```python
from build123d import *

# Parameters (mm, degrees)
SKETCH2_W           = 304.8
SKETCH2_H           = 17.78
BOSS_EXTRUDE1_DEPTH = 152.4
SKETCH3_W           = 121.604136641
SKETCH3_H           = 12.7
CUT_EXTRUDE1_DEPTH  = 305.8
CUT_EXTRUDE2_DEPTH  = 203.2
BOSS_EXTRUDE6_DEPTH = 63.5
BOSS_EXTRUDE8_DEPTH = 76.2
BOSS_EXTRUDE9_DEPTH = 69.163311
CUT_EXTRUDE4_REACH  = 230.6
SKETCH14_W          = 31.75
SKETCH14_H          = 203.2
CUT_EXTRUDE5_DEPTH  = 116.484487595
SKETCH15_W          = 69.163311332
SKETCH15_H          = 50.8
CUT_EXTRUDE6_DEPTH  = 12.7


with BuildPart() as part:
    # Sketch2 → Boss-Extrude1 (new body)
    with BuildSketch(Plane.XY):
        with Locations((152.4, 8.89)):
            Rectangle(SKETCH2_W, SKETCH2_H)
    extrude(amount=BOSS_EXTRUDE1_DEPTH)

    # Sketch3 → Cut-Extrude1 (cut, through all)
    with BuildSketch(Plane(origin=(304.8, 0, 0), x_dir=(0, 0, -1), z_dir=(1, 0, 0))):
        Polygon((-152.4, 17.78), (-152.4, 0), (-121.604136641, 17.78), align=None)
        with Locations((-60.802068321, 11.43)):
            Rectangle(SKETCH3_W, SKETCH3_H)
    extrude(amount=-CUT_EXTRUDE1_DEPTH, mode=Mode.SUBTRACT)

    # Sketch4 → Cut-Extrude2 (cut)
    with BuildSketch(Plane(origin=(0, 5.08, 0), x_dir=(1, 0, 0), z_dir=(0, 1, 0))):
        Polygon((0, 0), (0, -112.812583018), (117.818344334, 0), align=None)
        Polygon((304.8, 0), (186.981655666, 0), (304.8, -112.812583018), align=None)
    extrude(amount=-CUT_EXTRUDE2_DEPTH, mode=Mode.SUBTRACT)

    # Sketch5 → Boss-Extrude6 (add)
    with BuildSketch(Plane(origin=(0, 5.08, 0), x_dir=(1, 0, 0), z_dir=(0, 1, 0))):
        Polygon((127, 0), (117.818344334, 0), (0, -112.812583018), (0, -121.604136641), (12.7, -121.604136641), align=None)
        Polygon((177.8, 0), (186.981655666, 0), (304.8, -112.812583018), (304.8, -121.604136641), (292.1, -121.604136641), align=None)
    extrude(amount=BOSS_EXTRUDE6_DEPTH)

    # Sketch8 → Boss-Extrude8 (add)
    with BuildSketch(Plane(origin=(0, 0, 0), x_dir=(-1, 0, 0), z_dir=(0, 0, -1))):
        Polygon((-186.981655666, 68.58), (-186.981655666, 0), (-117.818344334, 0), (-117.818344334, 68.58), (-127, 68.58), (-127, 5.08), (-177.8, 5.08), (-177.8, 68.58), align=None)
    extrude(amount=BOSS_EXTRUDE8_DEPTH)

    # Sketch10 → Boss-Extrude9 (add)
    with BuildSketch(Plane(origin=(186.981655666, 0, 0), x_dir=(0, 0, -1), z_dir=(1, 0, 0))):
        Polygon((6.35, 0), (0, 0), (127, 219.970452561), (133.35, 219.970452561), align=None)
    extrude(amount=-BOSS_EXTRUDE9_DEPTH)

    # Cut-Extrude4: up to this face of the body (flat: up to its plane)
    cut_extrude4_end = Plane(part.part.faces().sort_by_distance((152.400000127, 118.969659324, -75.037164836))[0])
    # Sketch12 → Cut-Extrude4 (cut, up to the picked face)
    with BuildSketch(Plane(origin=(0, 0, -76.2), x_dir=(-1, 0, 0), z_dir=(0, 0, -1)), mode=Mode.PRIVATE) as cut_extrude4_sk1:
        Polygon((-186.981655666, 0), (-186.981655666, 68.58), (-177.8, 68.58), (-177.8, 5.08), (-127, 5.08), (-127, 68.58), (-117.818344334, 68.58), (-117.818344334, 0), align=None)
    cut_extrude4_tool1 = split(extrude(cut_extrude4_sk1.sketch, amount=-CUT_EXTRUDE4_REACH, mode=Mode.PRIVATE), bisect_by=cut_extrude4_end, keep=Keep.BOTH, mode=Mode.PRIVATE)
    add(cut_extrude4_tool1.solids().sort_by_distance((186.007655, 34.29, -76.2))[0], mode=Mode.SUBTRACT)

    # Sketch14 → Cut-Extrude5 (cut, through all)
    with BuildSketch(Plane(origin=(0, 0, 0), x_dir=(1, 0, 0), z_dir=(0, 0.5, 0.866025404))):
        with Locations((152.4, 180.789362922)):
            Rectangle(SKETCH14_W, SKETCH14_H)
    extrude(amount=-CUT_EXTRUDE5_DEPTH, mode=Mode.SUBTRACT)

    # Sketch15 → Cut-Extrude6 (cut)
    with BuildSketch(Plane(origin=(0, 0, 0), x_dir=(1, 0, 0), z_dir=(0, 0.5, 0.866025404))):
        with Locations((152.4, 231.775)):
            Rectangle(SKETCH15_W, SKETCH15_H)
    extrude(amount=-CUT_EXTRUDE6_DEPTH, mode=Mode.SUBTRACT)


solid = part.part
```
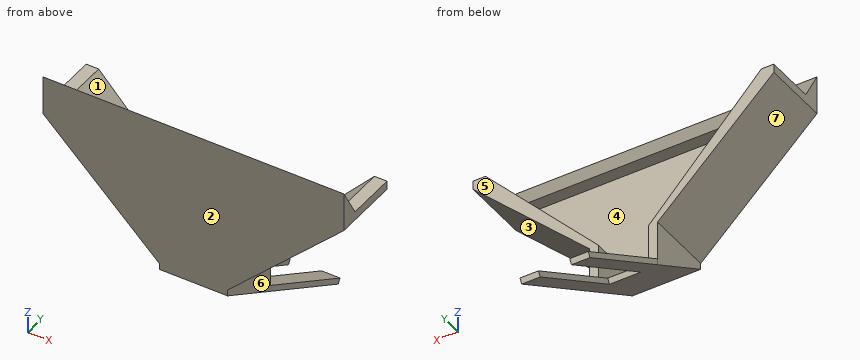
Model file for the job. Use its own axes, mm. Face numbers are marked on the shaded views. A direction names the side the tool comes from. Round coordinates to 2 decimals unless told otherwise and drop trailing zeros. Write each loop counter-clockwise with the first axis right and the second up, starting at its lowest first coordinate (ties: lowest second). Pieces come first, ordered by that corner, then holes. Notation, with made-up numbers: M 10.25,-15 L 27.25,-15 A25 ccw 27.25,-3 Z; hole C -14.5,41 d3. An arc over 180 degrees is marked long. Put each result on its own line as item: value.
Item 1: Mould opens along Z. For the marked faces 1, 2, 3 and 4 say: +Z half, -Z half, draft (parallel to the pull), parting line (faces both ways), or undercut.
Responses:
face 1: undercut
face 2: draft
face 3: -Z half
face 4: undercut
Item 2: Cut at D-D (y = 35). List the corners of the cut face in (x, z).
Responses:
outline: M 0,112.81 L 117.82,0 L 117.82,-26.56 L 186.98,-26.56 L 186.98,0 L 304.8,112.81 L 304.8,121.6 L 292.1,121.6 L 177.8,0 L 177.8,-20.21 L 127,-20.21 L 127,0 L 12.7,121.6 L 0,121.6 Z
Item 3: Flat gauge pins, fed straight in: P1, Ø1, axis at x = 61.5, y = 24, coming from the +Z side; P2, Ø1, axis at y = 53, z = 6, coming from the +X side; P3, Ø3, axis at x = 132, y = 109, coming from the -Z side; P4, Ø10, axis at x = 66, y = 77, coming from the +Z side. Where does each tip first touch, or does it go through?
Responses:
P1: z = 70.22
P2: x = 193.77
P3: z = -70.15
P4: through
Item 4: Cut at A-A (y = 124.5). List the corners of the cut face in (x, z) (3 decimals).
Responses:
outline: M 117.818,-78.23 L 136.525,-78.23 L 136.525,-71.88 L 117.818,-71.88 Z; M 168.275,-78.23 L 186.982,-78.23 L 186.982,-71.88 L 168.275,-71.88 Z
Item 5: Cut at B-B (z = 65). List the corners of the cut face in (x, y).
Responses:
outline: M 49.93,0 L 254.87,0 L 254.87,68.58 L 238.9,68.58 L 238.9,5.08 L 65.9,5.08 L 65.9,68.58 L 49.93,68.58 Z
Item 6: Tool access for the marked faces 5, 6 and 7: list every direction of +Z, -Z, +X, -X, +Y, -Y with a clear straight run to the whole face (end or side of a thin tool).
Responses:
face 5: +Z, +X, -X, +Y
face 6: -Z, +X, +Y, -Y
face 7: -Z, -X, +Y, -Y
Item 7: Probe L1, parallel to X at y = 46, z = -9; L2, parallel to X at y = 21, z = 65; L3, parallel to Y at x = 201, z = 60.5. List the from-to ranges inside material, lowest first. Write a range as from..to.
Responses:
L1: 117.82..127, 177.8..186.98
L2: 49.93..65.9, 238.9..254.87
L3: 0..5.08
Item 8: Cut at C-C (x = 58). List the corners of the cut face in (y, z), and give its area (3 significant figures).
Responses:
outline: M 0,57.28 L 68.58,57.28 L 68.58,73.41 L 5.08,73.41 L 5.08,121.6 L 17.78,121.6 L 0,152.4 Z
area: 1,620 mm²
